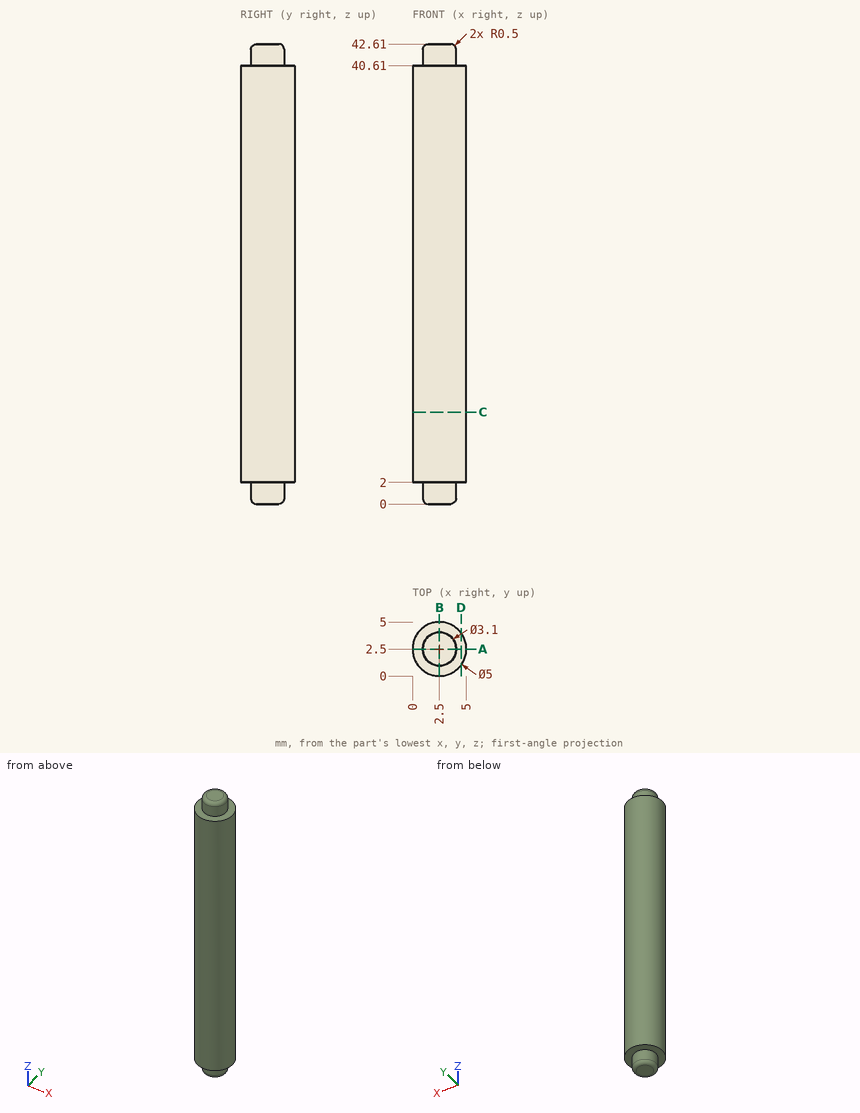
Study the drawing (mm; zero at the part's minimum x, y, z) and answer. Give positions to 0.01 mm unless a question says otherwise; leave off trailing zeros. Write each loop counter-clockwise with the first axis right and the second up, starting at its lowest first coordinate (ties: lowest second). Pieces come first, ordered by that corner, then holes.
(1) The part is cut by section D-D on x = 4.5. Write down the section's boundary in (y, z).
Final values:
outline: (1, 2) - (4, 2) - (4, 40.61) - (1, 40.61) - close
(2) The part is cut by section C-C on z = 8.5. Write down the section's boundary in (x, y), plus the area to 3 significant figures.
Final values:
outline: circle Ø5 at (2.5, 2.5)
area: 19.6 mm2
(3) Straight lines are drawn through the part: line 1 (Z direction, x = 1.4, y = 0.65); line 2 (Y direction, x = 2.6, z = 26); line 3 (X direction, y = 4.2, z = 39). For each, find the intervals that lie inside material, in ascending order.
Final values:
line 1: z = 2 to 40.61
line 2: y = 0 to 5
line 3: x = 0.67 to 4.33
(4) Flat-ended cylindrical pins translate along their axes: pin 1 Ø2 at (x, z) = (1, 25) entering from -Y; pin 2 Ø2 at (x, z) = (1.5, 12) entering from -Y; pin 3 Ø1 at (x, y) = (1.5, 4) entering from -Z. Find the tip coordinate at first contact, or state that the pin passes through.
Final values:
pin 1: stops at y = 0.05
pin 2: stops at y = 0
pin 3: stops at z = 0.07
(5) The part is cut by section A-A on y = 2.5. Write down the section's boundary in (x, z).
Final values:
outline: (0, 2) - (0.95, 2) - (0.95, 0.5) arc R0.5 ccw to (1.45, 0) - (3.55, 0) arc R0.5 ccw to (4.05, 0.5) - (4.05, 2) - (5, 2) - (5, 40.61) - (4.05, 40.61) - (4.05, 42.11) arc R0.5 ccw to (3.55, 42.61) - (1.45, 42.61) arc R0.5 ccw to (0.95, 42.11) - (0.95, 40.61) - (0, 40.61) - close
